```python
from build123d import *

# Parameters (mm, degrees)
CYLINDER082_R          = 0.5
CYLINDER082_DEPTH      = 0.01
BOX179_W               = 4.5
BOX179_H               = 5.5
BOX179_DEPTH           = 0.5
CUT088_PLACEMENT_ANGLE = 122


with BuildPart() as cylinder082:
    # Cylinder082 → Cylinder082 (new body)
    with BuildSketch(Plane(origin=(1, 4.5, 0.49), x_dir=(1, 0, 0), z_dir=(0, 0, 1))):
        Circle(CYLINDER082_R)
    extrude(amount=CYLINDER082_DEPTH)


with BuildPart() as obj1:
    # Box179 → Box179 (new body)
    with BuildSketch(Plane.XY):
        with Locations((2.25, 2.75)):
            Rectangle(BOX179_W, BOX179_H)
    extrude(amount=BOX179_DEPTH)

    # Cut088: cut Cylinder082
    add(cylinder082.part, mode=Mode.SUBTRACT)


with BuildPart() as obj1_1:
    # Cut088 placement: moved
    add(obj1.part.moved(Location((-9.677147, 22.819562, 2.79))).rotate(Axis((-9.677147, 22.819562, 2.79), (0, 0, -1)), CUT088_PLACEMENT_ANGLE))


solid = obj1_1.part
```
CAD build for the part. Positions are in the model's coordinates, mm. Round coordinates to 2 decimals unless told otherwise and drop trailing zeros. Write each loop counter-clockwise with the first axis right and the second up, starting at its lowest first coordinate (ties: lowest second). Pieces come first, ordered by that corner, then holes. Notation, with made-up numbers: M 36.25,-34.5 L 52.25,-34.5 A20 ccw 52.25,-25.5 Z; hole C -14.5,64.5 d7. An arc over 180 degrees is marked long. One line per question, with ' | ' between items.
1. Cut at B-B on z = 3.1. Write the cut outline in (x, y) (3 decimals).
Working result:
outline: M -12.062,19.003 L -7.398,16.089 L -5.013,19.905 L -9.677,22.82 Z
2. Mould opens along Y. For faces 1 (the flat face through (-6.4, 19.6, 3.28)), 2 (the flat face through (-8, 19, 2.79)), 3 (the flat face through (-7.378, 21.383, 3.036)) say: pulls with the +Y half, pulls with the -Y half, needs draft (parallel to the pull), parting line crosses it, or undercut.
Working result:
face 1: undercut | face 2: needs draft | face 3: pulls with the +Y half
3. Probe L1, parallel to Z at x = -6.5, y = 19.75; L2, parallel to Y at x = -8.25, z = 3.05; L3, parallel to X at y = 20.25, z = 2.9. List the from-to ranges inside material, lowest first. Write a range as from..to.
Working result:
L1: 2.79..3.28 | L2: 16.62..21.93 | L3: -11.28..-5.56
4. Cut at D-D on x = -5.75. Write the cut outline in (y, z).
Working result:
outline: M 18.73,2.79 L 20.37,2.79 L 20.37,3.29 L 18.73,3.29 Z
